Check sheet for the modelled part. Datum: model origin and axes. Units: mm. Round coordinates to 2 decimals unless told otherwise and drop trailing zeros. Order: outer loops, then holes, each group sorted by start corner. A loop starts at its lowest first (then second) coordinate and runs counter-clockwise, first axis right, second up. Notation, with made-up numbers: (36.5, 12) -> (63.5, 12) arc R21 cw to (63.5, 44) -> close; hole circle Ø8 at (82, -11). An arc over 180 degrees is marked (long way). Answer in a Markdown table with one row per item.
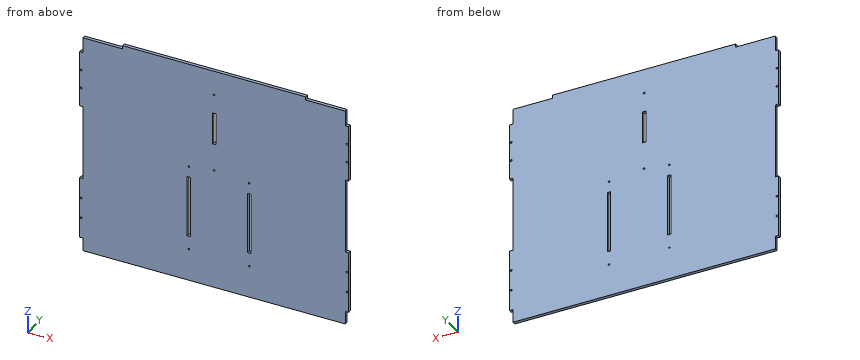
```python
from build123d import *

# Parameters (mm, degrees)
SKETCH1_W             = 490
SKETCH1_H             = 411.98
BOSS_EXTRUDE1_DEPTH   = 6
SKETCH2_W             = 78.33333333
SKETCH2_H             = 6
SKETCH2_W_2           = 6
SKETCH2_H_2           = 137.326666666
CUT_EXTRUDE1_DEPTH    = 12
SKETCH4_W             = 6
SKETCH4_H             = 24
SKETCH4_H_2           = 27.996666667
CUT_EXTRUDE2_DEPTH    = 12
SKETCH6_W             = 6
SKETCH6_H             = 58.97
CUT_EXTRUDE3_DEPTH    = 641.20584221
M3_CLEARANCE_HOLE1_D  = 3.4
F_3_0MM_DOWEL_HOLE1_D = 3
CUT_EXTRUDE4_REACH    = 642.206
SKETCH11_W            = 6
SKETCH11_H            = 113


with BuildPart() as part:
    # Sketch1 → Boss-Extrude1 (new body)
    with BuildSketch(Plane(origin=(0, 0, 0), x_dir=(1, 0, 0), z_dir=(0, 1, 0))):
        with Locations((245, 205.99)):
            Rectangle(SKETCH1_W, SKETCH1_H)
    extrude(amount=BOSS_EXTRUDE1_DEPTH)

    # Sketch2 → Cut-Extrude1 (cut)
    with BuildSketch(Plane(origin=(0, 6, 0), x_dir=(1, 0, 0), z_dir=(0, 1, 0))):
        with Locations((39.166666665, 3)):
            Rectangle(SKETCH2_W, SKETCH2_H)
        with Locations((450.833333335, 3)):
            Rectangle(SKETCH2_W, SKETCH2_H)
        with Locations((3, 205.99)):
            Rectangle(SKETCH2_W_2, SKETCH2_H_2)
        with Locations((487, 205.99)):
            Rectangle(SKETCH2_W_2, SKETCH2_H_2)
    extrude(amount=-CUT_EXTRUDE1_DEPTH, mode=Mode.SUBTRACT)

    # Sketch4 → Cut-Extrude2 (cut)
    with BuildSketch(Plane(origin=(0, 6, 0), x_dir=(1, 0, 0), z_dir=(0, 1, 0))):
        with Locations((3, 399.98)):
            Rectangle(SKETCH4_W, SKETCH4_H)
        with Locations((487, 399.98)):
            Rectangle(SKETCH4_W, SKETCH4_H)
        with Locations((487, 19.998333333)):
            Rectangle(SKETCH4_W, SKETCH4_H_2)
        with Locations((3, 19.998333333)):
            Rectangle(SKETCH4_W, SKETCH4_H_2)
    extrude(amount=-CUT_EXTRUDE2_DEPTH, mode=Mode.SUBTRACT)

    # Sketch6 → Cut-Extrude3 (cut, through all)
    with BuildSketch(Plane(origin=(0, 6, 0), x_dir=(1, 0, 0), z_dir=(0, 1, 0))):
        with Locations((245, 109.485)):
            Rectangle(SKETCH6_W, SKETCH6_H)
    extrude(amount=-CUT_EXTRUDE3_DEPTH, mode=Mode.SUBTRACT)

    # M3 Clearance Hole1 (through all)
    with Locations(Plane(origin=(0, 6, 0), x_dir=(1, 0, 0), z_dir=(0, 1, 0))):
        with Locations((3, 350.203333333), (3, 312.43), (3, 102.883333333), (3, 68.44), (487, 350.203333333), (487, 312.43), (487, 102.883333333), (487, 68.44), (245, 188.97), (245, 45)):
            Hole(M3_CLEARANCE_HOLE1_D / 2)

    # Ø3.0mm Dowel Hole1 (through all)
    with Locations(Plane(origin=(0, 6, 0), x_dir=(1, 0, 0), z_dir=(0, 1, 0))):
        with Locations((309, 352.98), (309, 194.98), (199, 352.98), (199, 194.98)):
            Hole(F_3_0MM_DOWEL_HOLE1_D / 2)

    # Sketch11 → Cut-Extrude4 (cut, up to next)
    with BuildSketch(Plane.XZ, mode=Mode.PRIVATE) as cut_extrude4_sk1:
        with Locations((309, -271.48)):
            Rectangle(SKETCH11_W, SKETCH11_H)
    cut_extrude4_tool1 = extrude(cut_extrude4_sk1.sketch, amount=-CUT_EXTRUDE4_REACH, mode=Mode.PRIVATE) & part.part
    # Sketch11 → Cut-Extrude4 (cut, up to next)
    with BuildSketch(Plane.XZ, mode=Mode.PRIVATE) as cut_extrude4_sk2:
        with Locations((199, -271.48)):
            Rectangle(SKETCH11_W, SKETCH11_H)
    cut_extrude4_tool2 = extrude(cut_extrude4_sk2.sketch, amount=-CUT_EXTRUDE4_REACH, mode=Mode.PRIVATE) & part.part
    add(cut_extrude4_tool1.solids().sort_by_distance((309, 0, -271.48))[0], mode=Mode.SUBTRACT)
    add(cut_extrude4_tool2.solids().sort_by_distance((199, 0, -271.48))[0], mode=Mode.SUBTRACT)


solid = part.part
```
(1) Section check C-C on y = 1.95. Give the number of separate pieces and of enclosed holes in the cut face, plus the area to 3 significant figures.
Solutions:
| item | result |
|---|---|
| separate pieces | 1 |
| enclosed holes | 17 |
| area | 197,000 mm^2 |
(2) Depth check by flat-ended pin: pin 1 Ø3 at (x, y) = (439.5, 3) entering from +Z; pin 2 Ø1.5 at (y, z) = (5, -206.5) entering from +X; pin 3 Ø1.8 at (x, y) = (488, 4.5) entering from -Z. Enter the tip coordinate at first touch or a pass-through.
Solutions:
| item | result |
|---|---|
| pin 1 | z = -6 |
| pin 2 | x = 484 |
| pin 3 | z = -387.98 |
(3) Scan lines: probe 1 along Z at (x, y) = (199, 2.2); probe 2 along Z at (x, y) = (3, 1.9); probe 3 along X at (y, z) = (1.1, -315). Record each from-to range of solid material in increasing order. Write a range as from..to.
Solutions:
| item | result |
|---|---|
| probe 1 | -411.98..-354.48, -351.48..-327.98, -214.98..-196.48, -193.48..0 |
| probe 2 | -387.98..-351.9, -348.5..-314.13, -310.73..-274.65, -137.33..-104.58, -101.18..-70.14, -66.74..-34 |
| probe 3 | 0..196, 202..306, 312..490 |
(4) Section check A-A on z = -321. Record the boundary of the cut face in (x, y).
Solutions:
| item | result |
|---|---|
| outline | (0, 0) -> (196, 0) -> (196, 6) -> (0, 6) -> close; (202, 0) -> (306, 0) -> (306, 6) -> (202, 6) -> close; (312, 0) -> (490, 0) -> (490, 6) -> (312, 6) -> close |
(5) Section check B-B on z = -27.5. Record the boundary of the cut face in (x, y).
Solutions:
| item | result |
|---|---|
| outline | (6, 0) -> (484, 0) -> (484, 6) -> (6, 6) -> close |
